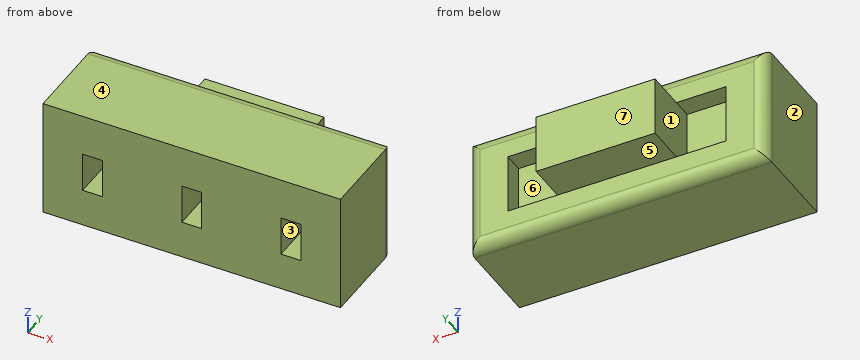
from build123d import *

# Parameters (mm, degrees)
SKETCH1_W           = 7.5
SKETCH1_H           = 3
BOSS_EXTRUDE1_DEPTH = 2.4
SKETCH2_W           = 3
SKETCH2_H           = 1.5
BOSS_EXTRUDE2_DEPTH = 1
SKETCH3_W           = 1.25
SKETCH3_H           = 1.5
CUT_EXTRUDE1_DEPTH  = 0.5
SKETCH4_W           = 0.5
SKETCH4_H           = 1
CUT_EXTRUDE2_DEPTH  = 1
FILLET1_R           = 0.3


with BuildPart() as part:
    # Sketch1 → Boss-Extrude1 (new body)
    with BuildSketch(Plane(origin=(0, 0, 0), x_dir=(1, 0, 0), z_dir=(0, 1, 0))):
        with Locations((-0.439685246, 1.166396104)):
            Rectangle(SKETCH1_W, SKETCH1_H)
    extrude(amount=BOSS_EXTRUDE1_DEPTH)

    # Sketch2 → Boss-Extrude2 (add)
    with BuildSketch(Plane(origin=(0, 2.4, 0), x_dir=(1, 0, 0), z_dir=(0, 1, 0))):
        with Locations((-0.439685246, 1.166396104)):
            Rectangle(SKETCH2_W, SKETCH2_H)
    extrude(amount=BOSS_EXTRUDE2_DEPTH)

    # Sketch3 → Cut-Extrude1 (cut)
    with BuildSketch(Plane(origin=(0, 2.4, 0), x_dir=(1, 0, 0), z_dir=(0, 1, 0))):
        with Locations((1.685314754, 1.166396104)):
            Rectangle(SKETCH3_W, SKETCH3_H)
        with Locations((-2.564685246, 1.166396104)):
            Rectangle(SKETCH3_W, SKETCH3_H)
    extrude(amount=-CUT_EXTRUDE1_DEPTH, mode=Mode.SUBTRACT)

    # Sketch4 → Cut-Extrude2 (cut)
    with BuildSketch(Plane.XZ):
        with Locations((2.060314754, -1.211874682)):
            Rectangle(SKETCH4_W, SKETCH4_H)
        with Locations((-0.439685246, -1.211874682)):
            Rectangle(SKETCH4_W, SKETCH4_H)
        with Locations((-2.939685246, -1.211874682)):
            Rectangle(SKETCH4_W, SKETCH4_H)
    extrude(amount=-CUT_EXTRUDE2_DEPTH, mode=Mode.SUBTRACT)

    # Fillet1
    fillet1_edges = [part.edges().sort_by_distance(p)[0] for p in [
        (3.310314754, 2.4, -1.166396104),
        (-0.439685246, 2.4, -2.666396104),
        (-4.189685246, 2.4, -1.166396104),
        (-0.439685246, 2.4, 0.333603896),
    ]]
    fillet(fillet1_edges, radius=FILLET1_R)


solid = part.part
Work out the finished part from the listing and answer in its coordinate system (mm). Face numbers are marked on the shaded views. A direction names the side the tool comes from. Round coordinates to 2 decimals unless told otherwise and drop trailing zeros. Order: outer loops, then holes, each group sorted by start corner. A loop starts at its lowest first (then second) coordinate and runs counter-clockwise, first axis right, second up. Notation, with made-up numbers: M -5,-40 L 16,-40 A22 cw 16,-14 Z; hole C 42.25,48.5 d5. An arc over 180 degrees is marked long. Put each result on its own line as item: value. Start each with the question number.
Q1. For a pull along Z with two mould halves and no side action, classify the marked faces 4, 5, 6 and 7 as pulls with the +Z half, pulls with the -Z half, needs draft (parallel to the pull), parting line crosses it, or undercut.
Q2. A tool of negligible diameter and unlimited length cuts with its end or side. For the marked faces 1, 2 and 3, from which of +Z, -Z, +X, -X, +Y, -Y can it reach the whole face along a straight path? Write none if from no direction.
Q3. Section B-B, the plane x = 0 is taken. Write down the section's boundary in (y, z).
Q4. Straight lines are drawn through the part: L1, parallel to X at y = 0.2, z = -1.35; L2, parallel to X at y = 2, z = -0.5; L3, parallel to Z at x = -0.5, y = 0.4. For each, find the intervals that lie inside material, in ascending order. Write a range as [from, to].
Q5. Section D-D, the plane y = 2 is taken. Write down the section's boundary in (x, z).
Q6. Section A-A, the plane y = 0.65 is taken. Write down the section's boundary in (x, z), and give its area (3 significant figures).
Q7. Section C-C, the plane z = -0.8 is taken. Write down the section's boundary in (x, y).
Findings below:
1. face 4: pulls with the +Z half
1. face 5: pulls with the -Z half
1. face 6: undercut
1. face 7: needs draft
2. face 1: +Y
2. face 2: +Z, -Z, -X, +Y, -Y
2. face 3: -Y
3. outline: M 0,-2.67 L 2.1,-2.67 A0.3 ccw 2.4,-2.37 L 2.4,-1.92 L 3.4,-1.92 L 3.4,-0.42 L 2.4,-0.42 L 2.4,0.03 A0.3 ccw 2.1,0.33 L 0,0.33 Z
4. L1: x = [-4.19, -3.19], [-2.69, -0.69], [-0.19, 1.81], [2.31, 3.31]
4. L2: x = [-4.19, -3.19], [-1.94, 1.06], [2.31, 3.31]
4. L3: z = [-2.67, -1.71], [-0.71, 0.33]
5. outline: M -4.19,-2.67 L 3.31,-2.67 L 3.31,0.33 L -4.19,0.33 Z; hole M -3.19,-1.92 L -1.94,-1.92 L -1.94,-0.42 L -3.19,-0.42 Z; hole M 1.06,-1.92 L 2.31,-1.92 L 2.31,-0.42 L 1.06,-0.42 Z
6. outline: M -4.19,-2.67 L 3.31,-2.67 L 3.31,0.33 L -4.19,0.33 Z; hole M -3.19,-1.71 L -2.69,-1.71 L -2.69,-0.71 L -3.19,-0.71 Z; hole M -0.69,-1.71 L -0.19,-1.71 L -0.19,-0.71 L -0.69,-0.71 Z; hole M 1.81,-1.71 L 2.31,-1.71 L 2.31,-0.71 L 1.81,-0.71 Z
6. area: 21.0 mm^2
7. outline: M -4.19,0 L -3.19,0 L -3.19,1 L -2.69,1 L -2.69,0 L -0.69,0 L -0.69,1 L -0.19,1 L -0.19,0 L 1.81,0 L 1.81,1 L 2.31,1 L 2.31,0 L 3.31,0 L 3.31,2.1 A0.3 ccw 3.01,2.4 L 2.31,2.4 L 2.31,1.9 L 1.06,1.9 L 1.06,3.4 L -1.94,3.4 L -1.94,1.9 L -3.19,1.9 L -3.19,2.4 L -3.89,2.4 A0.3 ccw -4.19,2.1 Z
